Model file for the job. Use its own axes, mm. Face numbers are marked on the shaded views. A direction names the side the tool comes from. Coordinates: 2 decimals unless noted, no trailing zeros. Loops run counter-clockwise (first coordinate to the right, second up) from the corner with the lowest first, then second, coordinate; pieces in that order, holes last.
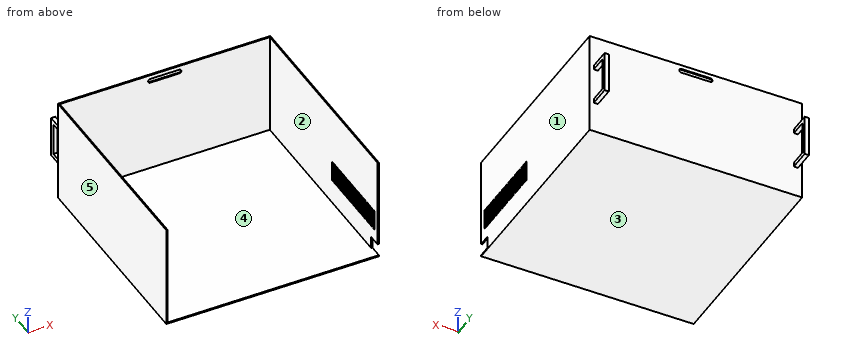
from build123d import *

# Parameters (mm, degrees)
ESBO_O1_W                = 512
ESBO_O1_H                = 505
RESSALTO_EXTRUS_O1_DEPTH = 500
ESBO_O2_W                = 522
ESBO_O2_H                = 510
CORTE_EXTRUS_O1_DEPTH    = 252.5
ESBO_O6_W                = 506
ESBO_O6_H                = 497
CORTE_EXTRUS_O4_DEPTH    = 249.5
ESBO_O7_W                = 30
ESBO_O7_H                = 30
CABO_DE_ALIMENTA_O_DEPTH = 5
ESBO_O9_W                = 50
ESBO_O9_H                = 5
CORTE_EXTRUS_O6_DEPTH    = 5
PASSAGEM_FILAMENTO_DEPTH = 5
ESBO_O69_W               = 10
ESBO_O69_H               = 100
AL_A_2_DEPTH             = 50
ESBO_O70_W               = 80
ESBO_O70_H               = 40
AL_A_2_2_DEPTH           = 10
ESBO_O72_W               = 10
ESBO_O72_H               = 100
AL_A_1_DEPTH             = 50
ESBO_O74_W               = 80
ESBO_O74_H               = 40
AL_A_1_2_DEPTH           = 10


with BuildPart() as part:
    # Esboço1 → Ressalto-extrusão1 (new body)
    with BuildSketch(Plane(origin=(0, 0, 0), x_dir=(1, 0, 0), z_dir=(0, 1, 0))):
        Rectangle(ESBO_O1_W, ESBO_O1_H)
    extrude(amount=RESSALTO_EXTRUS_O1_DEPTH)

    # Esboço2 → Corte-extrusão1 (cut)
    with BuildSketch(Plane.XY.offset(252.5)):
        with Locations((0, 250)):
            Rectangle(ESBO_O2_W, ESBO_O2_H)
    extrude(amount=-CORTE_EXTRUS_O1_DEPTH, mode=Mode.SUBTRACT)

    # Esboço6 → Corte-extrusão4 (cut)
    with BuildSketch(Plane.XY):
        with Locations((0, 248.5)):
            Rectangle(ESBO_O6_W, ESBO_O6_H)
    extrude(amount=-CORTE_EXTRUS_O4_DEPTH, mode=Mode.SUBTRACT)

    # Esboço7 → Cabo de alimentação (cut)
    with BuildSketch(Plane(origin=(256, 0, 0), x_dir=(0, 0, -1), z_dir=(1, 0, 0))):
        with Locations((234.5, 15)):
            Rectangle(ESBO_O7_W, ESBO_O7_H)
    extrude(amount=-CABO_DE_ALIMENTA_O_DEPTH, mode=Mode.SUBTRACT)

    # Esboço9 → Corte-extrusão6 (cut)
    with BuildSketch(Plane(origin=(256, 0, 0), x_dir=(0, 0, -1), z_dir=(1, 0, 0))):
        with Locations((164.5, 17.5)):
            Rectangle(ESBO_O9_W, ESBO_O9_H)
        with Locations((164.5, 27.5)):
            Rectangle(ESBO_O9_W, ESBO_O9_H)
        with Locations((164.5, 47.5)):
            Rectangle(ESBO_O9_W, ESBO_O9_H)
        with Locations((164.5, 37.5)):
            Rectangle(ESBO_O9_W, ESBO_O9_H)
        with Locations((164.5, 67.5)):
            Rectangle(ESBO_O9_W, ESBO_O9_H)
        with Locations((164.5, 77.5)):
            Rectangle(ESBO_O9_W, ESBO_O9_H)
        with Locations((164.5, 87.5)):
            Rectangle(ESBO_O9_W, ESBO_O9_H)
        with Locations((164.5, 57.5)):
            Rectangle(ESBO_O9_W, ESBO_O9_H)
        with Locations((164.5, 107.5)):
            Rectangle(ESBO_O9_W, ESBO_O9_H)
        with Locations((164.5, 157.5)):
            Rectangle(ESBO_O9_W, ESBO_O9_H)
        with Locations((164.5, 117.5)):
            Rectangle(ESBO_O9_W, ESBO_O9_H)
        with Locations((164.5, 167.5)):
            Rectangle(ESBO_O9_W, ESBO_O9_H)
        with Locations((164.5, 127.5)):
            Rectangle(ESBO_O9_W, ESBO_O9_H)
        with Locations((164.5, 97.5)):
            Rectangle(ESBO_O9_W, ESBO_O9_H)
        with Locations((164.5, 147.5)):
            Rectangle(ESBO_O9_W, ESBO_O9_H)
        with Locations((164.5, 137.5)):
            Rectangle(ESBO_O9_W, ESBO_O9_H)
        with Locations((164.5, 177.5)):
            Rectangle(ESBO_O9_W, ESBO_O9_H)
        with Locations((164.5, 187.5)):
            Rectangle(ESBO_O9_W, ESBO_O9_H)
        with Locations((164.5, 207.5)):
            Rectangle(ESBO_O9_W, ESBO_O9_H)
        with Locations((164.5, 197.5)):
            Rectangle(ESBO_O9_W, ESBO_O9_H)
    extrude(amount=-CORTE_EXTRUS_O6_DEPTH, mode=Mode.SUBTRACT)

    # Esboço68 → Passagem Filamento (cut)
    with BuildSketch(Plane(origin=(0, 500, 0), x_dir=(1, 0, 0), z_dir=(0, 1, 0))):
        with BuildLine():
            Line((-35, 20), (35, 20))
            ThreePointArc((35, 20), (40, 15), (35, 10))
            Line((35, 10), (-35, 10))
            ThreePointArc((-35, 10), (-40, 15), (-35, 20))
        make_face()
    extrude(amount=-PASSAGEM_FILAMENTO_DEPTH, mode=Mode.SUBTRACT)

    # Esboço69 → Al_a - 2 (add)
    with BuildSketch(Plane(origin=(0, 500, 0), x_dir=(1, 0, 0), z_dir=(0, 1, 0))):
        with Locations((-241, 126.25)):
            Rectangle(ESBO_O69_W, ESBO_O69_H)
    extrude(amount=AL_A_2_DEPTH)

    # Esboço70 → Al_a _2 2 (cut)
    with BuildSketch(Plane.ZY.offset(246)):
        with Locations((-126.25, 520)):
            Rectangle(ESBO_O70_W, ESBO_O70_H)
    extrude(amount=-AL_A_2_2_DEPTH, mode=Mode.SUBTRACT)

    # Esboço72 → Al_a - 1 (add)
    with BuildSketch(Plane(origin=(531.113648875, 500, -10.670910915), x_dir=(1, 0, 0), z_dir=(0, 1, 0))):
        with Locations((-290.113648875, 115.579089085)):
            Rectangle(ESBO_O72_W, ESBO_O72_H)
    extrude(amount=AL_A_1_DEPTH)

    # Esboço74 → Al_a _1 2 (cut)
    with BuildSketch(Plane(origin=(236, 0, -10.670910915), x_dir=(0, 0, 1), z_dir=(-1, 0, 0))):
        with Locations((-115.579089085, 520)):
            Rectangle(ESBO_O74_W, ESBO_O74_H)
    extrude(amount=-AL_A_1_2_DEPTH, mode=Mode.SUBTRACT)


solid = part.part
Q1. Drill centre lines: line 1 (X direction, y = 365, z = -114); line 2 (X direction, y = 519.5, z = -81.5); line 3 (Y direction, x = -110.5, z = -145.5). Where is each one in solid material? Low to high.
Answers:
line 1: x = -256 to -253, 253 to 256
line 2: x = -246 to -236, 236 to 246
line 3: y = 497 to 500
Q2. Slice it at C-C (y = 243). List the corners of the cut face in (x, z), and give its area (3 significant figures).
Answers:
outline: (-256, -252.5) - (256, -252.5) - (256, 0) - (253, 0) - (253, -249.5) - (-253, -249.5) - (-253, 0) - (-256, 0) - close
area: 3,030 mm2
Q3. Mould opens along X. For the marked faces 3, 4 and 5 say: +X half, -X half, draft (parallel to the pull), parting line (faces both ways), or undercut.
Answers:
face 3: draft
face 4: undercut
face 5: -X half
Q4. Slice it at B-B (z = -130.5). List the corners of the cut face in (x, y), and give its area (3 significant figures).
Answers:
outline: (-256, 0) - (-253, 0) - (-253, 497) - (253, 497) - (253, 0) - (256, 0) - (256, 500) - (-256, 500) - close; (-246, 540) - (-236, 540) - (-236, 550) - (-246, 550) - close; (236, 540) - (246, 540) - (246, 550) - (236, 550) - close
area: 4,720 mm2
Q5. Flat gauge pins, fed straight in: P1, Ø1.5, axis at x = 73, z = -119, coming from the -Y side; P2, Ø5, axis at x = 243, y = 536, coming from the +Z side; P3, Ø12, axis at x = 149.5, y = 79.5, coming from the +Z side. Where does each tip first touch, or does it go through?
Answers:
P1: stops at y = 497
P2: stops at z = -76.25
P3: stops at z = -249.5
Q6. Slice it at D-D (z = -158.5). Count the separate pieces of the cut face and the enclosed holes in it, and give its area (3 significant figures).
Answers:
separate pieces: 23
enclosed holes: 0
area: 4,420 mm2
Q7. Slice it at A-A (x = -10). List the corners of the cut face in (y, z), and give its area (3 significant figures).
Answers:
outline: (0, -252.5) - (500, -252.5) - (500, -20) - (497, -20) - (497, -249.5) - (0, -249.5) - close; (497, -10) - (500, -10) - (500, 0) - (497, 0) - close
area: 2,220 mm2
Q8. Which spindle directions (+Z, -Z, +X, -X, +Y, -Y) get a long thin tool onto all of the face, cutting with end or side? Do the marked faces 1 and 2. Say none if no direction does.
Answers:
face 1: +Z, -Z, +X, +Y, -Y
face 2: +Z, -Y
